CAD build for the part. Positions are in the model's coordinates, mm. Face numbers are marked on the shaded views. A direction names the side the tool comes from. Round coordinates to 2 decimals unless told otherwise and drop trailing zeros. Loops run counter-clockwise (first coordinate to the right, second up) from the corner with the lowest first, then second, coordinate; pieces in that order, holes last. Notation, with made-up numbers: M 19,-18.5 L 45,-18.5 A33 cw 45,11.5 Z; hole C 29.25,30 d1. An arc over 180 degrees is marked long. One line per item, written item: value. Start each with the question number.
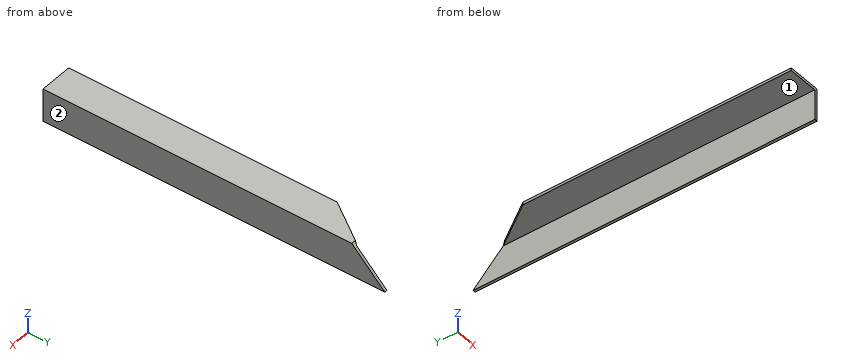
from build123d import *

# Parameters (mm, degrees)
F1_DEPTH = 787.4
F3_DEPTH = 76.2
F5_DEPTH = 25.4
F7_DEPTH = 25.4


with BuildPart() as f1:
    # F0 (on Front) → F1 (new body)
    with BuildSketch(Plane.XZ):
        Polygon((31.75, -38.1), (38.1, -38.1), (38.1, 38.1), (-38.1, 38.1), (-38.1, 31.75), (31.75, 31.75), align=None)
    extrude(amount=F1_DEPTH)

    # F2 (on face) → F3 (cut)
    with BuildSketch(Plane.YZ.offset(38.1)):
        Polygon((-76.2, 38.1), (0, -38.1), (0, 38.1), align=None)
    extrude(amount=-F3_DEPTH, mode=Mode.SUBTRACT)

    # F4 (on face) → F5 (cut)
    with BuildSketch(Plane.XY.offset(38.1)):
        Polygon((-38.1, -169.606138), (27.303682, -76.2), (-38.1, -76.2), align=None)
    extrude(amount=-F5_DEPTH, mode=Mode.SUBTRACT)

    # F6 (on face) → F7 (cut)
    with BuildSketch(Plane(origin=(0, 0, 31.75), x_dir=(1, 0, 0), z_dir=(0, 0, -1))):
        Polygon((-38.1, 69.85), (31.75, 69.85), (27.303682, 76.2), (-38.1, 76.2), align=None)
    extrude(amount=-F7_DEPTH, mode=Mode.SUBTRACT)


solid = f1.part
(1) Slice it at C-C, the plane x = -15.5. List the corners of the cut face in (y, z).
(2) Which spindle directions (+Z, -Z, +X, -X, +Y, -Y) get a long thin tool onto all of the face, cutting with end or side? Do the marked faces 1 and 2. Say none if no direction does.
(3) Slice it at B-B, the plane z = 13.5. List the corners of the cut face in (x, y), and give its area (3 significant figures).
(4) Probe L1, parallel to X at y = -540.5, z = -26; L2, parallel to Y at x = -25.5, z = 35. List the from-to ranges inside material, lowest first.
(5) Flat gauge pins, fed straight in: P1, Ø21, axis at x = -15.5, y = -454.5, coming from the -Z side; P2, Ø5, axis at x = 13.5, z = 28, coming from the +Y side. Where does each tip first touch, or does it go through?
(6) Slice it at A-A, the plane y = -589.5. List the corners of the cut face in (x, z), and give its area (3 significant figures).
Check result:
1. outline: M -787.4,31.75 L -137.33,31.75 L -137.33,38.1 L -787.4,38.1 Z
2. face 1: -Z, -X, +Y, -Y
2. face 2: +Z, -Z, +X, +Y, -Y
3. outline: M 31.75,-787.4 L 38.1,-787.4 L 38.1,-51.6 L 31.75,-51.6 Z
3. area: 4,670 mm^2
4. L1: x = 31.75 to 38.1
4. L2: y = -787.4 to -151.61
5. P1: stops at z = 31.75
5. P2: passes through
6. outline: M -38.1,31.75 L 31.75,31.75 L 31.75,-38.1 L 38.1,-38.1 L 38.1,38.1 L -38.1,38.1 Z
6. area: 927 mm^2
